```python
from build123d import *

# Parameters (mm, degrees)
F1_DEPTH = 9
F3_DEPTH = 9.001
F4_W     = 61.952739
F4_H     = 154.044632
F5_DEPTH = 9.001
F4_W_2   = 66.138744
F4_H_2   = 156.55623
F6_DEPTH = 9.001


with BuildPart() as f1:
    # F0 (on Top) → F1 (new body)
    with BuildSketch(Plane.XY):
        Polygon((143.506287, 346.454825), (-143.506287, 346.454825), (-346.454825, 143.506287), (-346.454825, -143.506287), (-143.506287, -346.454825), (143.506287, -346.454825), (346.454825, -143.506287), (346.454825, 143.506287), align=None)
    extrude(amount=F1_DEPTH)

    # F2 (on face) → F3 (cut, through all)
    with BuildSketch(Plane.XY.offset(9)):
        Polygon((346.454825, -143.506287), (-346.454825, -143.506287), (-143.506287, -346.454825), (143.506287, -346.454825), align=None)
    extrude(amount=-F3_DEPTH, mode=Mode.SUBTRACT)

    # F4 (on face) → F5 (cut, through all)
    with BuildSketch(Plane.XY.offset(9)):
        with Locations((-280.736581, 22.30238)):
            Rectangle(F4_W, F4_H)
    extrude(amount=-F5_DEPTH, mode=Mode.SUBTRACT)

    # F4 (on face) → F6 (cut, through all)
    with BuildSketch(Plane.XY.offset(9)):
        with Locations((278.931022, 23.558179)):
            Rectangle(F4_W_2, F4_H_2)
    extrude(amount=-F6_DEPTH, mode=Mode.SUBTRACT)


solid = f1.part
```
Check sheet for the modelled part. Datum: model origin and axes. Units: mm. Give positions to 0.01 mm unless a question says otherwise; leave off trailing zeros. Loops run counter-clockwise (first coordinate to the right, second up) from the corner with the lowest first, then second, coordinate; pieces in that order, holes last. Notation, with made-up numbers: M -15.5,58 L -9.5,58 A12 ccw -9.5,69 Z; hole C -34,-24.75 d2. An arc over 180 degrees is marked long. Answer in a Markdown table with one row per item.
1) Cross-section at B-B (z = 1.5). Enter the section's corners in (x, y), plus the area to 3 significant figures.
Solutions:
| item | result |
|---|---|
| outline | M -346.45,-143.51 L 346.45,-143.51 L 346.45,143.51 L 143.51,346.45 L -143.51,346.45 L -346.45,143.51 Z; hole M -311.71,-54.72 L -249.76,-54.72 L -249.76,99.32 L -311.71,99.32 Z; hole M 245.86,-54.72 L 312,-54.72 L 312,101.84 L 245.86,101.84 Z |
| area | 278,000 mm^2 |
2) Depth check by flat-ended pin: pin 1 (5 mm diameter, centred on x = 246, z = 2, fed in from +Y); pin 2 (4 mm diameter, centred on x = -251, z = 2, fed in from +Y). Enter the tip coordinate at first touch or a pass-through.
Solutions:
| item | result |
|---|---|
| pin 1 | stops at y = 246.46 |
| pin 2 | stops at y = 240.96 |
3) Cross-section at C-C (x = -279). Enter the section's corners in (y, z), plus the area to 3 significant figures.
Solutions:
| item | result |
|---|---|
| outline | M -143.51,0 L -54.72,0 L -54.72,9 L -143.51,9 Z; M 99.32,0 L 210.96,0 L 210.96,9 L 99.32,9 Z |
| area | 1,800 mm^2 |
4) Cross-section at A-A (y = 3.5). Enter the section's corners in (x, z).
Solutions:
| item | result |
|---|---|
| outline | M -346.45,0 L -311.71,0 L -311.71,9 L -346.45,9 Z; M -249.76,0 L 245.86,0 L 245.86,9 L -249.76,9 Z; M 312,0 L 346.45,0 L 346.45,9 L 312,9 Z |
5) Cross-section at D-D (x = 278). Enter the section's corners in (y, z), plus the area to 3 significant figures.
Solutions:
| item | result |
|---|---|
| outline | M -143.51,0 L -54.72,0 L -54.72,9 L -143.51,9 Z; M 101.84,0 L 211.96,0 L 211.96,9 L 101.84,9 Z |
| area | 1,790 mm^2 |
6) Thickness scan on line 1 (X direction, y = -38, z = 4); line 2 (Y direction, x = -250.5, z = 1.75); line 3 (Y direction, x = 311, z = 6). Record the ranges inside material, lowest first.
Solutions:
| item | result |
|---|---|
| line 1 | x = -346.45 to -311.71, -249.76 to 245.86, 312 to 346.45 |
| line 2 | y = -143.51 to -54.72, 99.32 to 239.46 |
| line 3 | y = -143.51 to -54.72, 101.84 to 178.96 |
